from build123d import *

# Parameters (mm, degrees)
EXTRUDE_1_DEPTH     = 2
SKETCH_2_R          = 2
EXTRUDE_2_DEPTH     = 7
CUT_EXTRUDE_2_DEPTH = 10


with BuildPart() as part:
    # 草图1 → 凸台-拉伸1 (new body)
    with BuildSketch(Plane(origin=(0, 0, 0), x_dir=(1, 0, 0), z_dir=(0, 1, 0))):
        with BuildLine():
            Line((-65, 5), (15, 5))
            ThreePointArc((15, 5), (20, 0), (15, -5))
            Line((15, -5), (-65, -5))
            ThreePointArc((-65, -5), (-70, 0), (-65, 5))
        make_face()
    extrude(amount=EXTRUDE_1_DEPTH)

    # 草图2 → 凸台-拉伸2 (add)
    with BuildSketch(Plane(origin=(0, 2, 0), x_dir=(1, 0, 0), z_dir=(0, 1, 0))):
        with Locations((15, 0)):
            Circle(SKETCH_2_R)
        with BuildLine():
            ThreePointArc((-63, 0), (-63.585786438, 1.414213562), (-65, 2))
            Line((-65, 2), (-65, -2))
            ThreePointArc((-65, -2), (-63.585786438, -1.414213562), (-63, 0))
        make_face()
        with BuildLine():
            Line((-65, -2), (-65, 2))
            ThreePointArc((-65, 2), (-67, 0), (-65, -2))
        make_face()
    extrude(amount=EXTRUDE_2_DEPTH)

    # 草图4 → 切除-拉伸2 (cut)
    with BuildSketch(Plane.XZ):
        with BuildLine():
            ThreePointArc((-23.015444247, 0.248069469), (-25.248069469, 1.984555753), (-26.984555753, -0.248069469))
            Line((-26.984555753, -0.248069469), (-23.015444247, 0.248069469))
        make_face()
        with BuildLine():
            Line((-23.015444247, 0.248069469), (-26.984555753, -0.248069469))
            ThreePointArc((-26.984555753, -0.248069469), (-24.875725117, -1.996135204), (-23, 0))
            ThreePointArc((-23, 0), (-23.003864796, 0.124274883), (-23.015444247, 0.248069469))
        make_face()
    extrude(amount=-CUT_EXTRUDE_2_DEPTH, mode=Mode.SUBTRACT)


solid = part.part
Build history of the part. All positions in model axes, mm. Coordinates: 2 decimals unless noted, no trailing zeros. Write each loop counter-clockwise with the first axis right and the second up, starting at its lowest first coordinate (ties: lowest second). Pieces come first, ordered by that corner, then holes.
(1) Pin check, flat tips, straight feed: pin 1 Ø2 at (x, y) = (-54.5, 3.5) entering from -Z; pin 2 Ø3 at (x, z) = (-30.5, 2.5) entering from +Y. Stop position of each tip, or through.
(2) Cut at B-B on y = 3.25. List the corners of the cut face in (x, z), and give its area (3 significant figures).
(3) Cut at A-A on x = -25. List the corners of the cut face in (y, z).
(4) Cut at C-C on x = -54. List the corners of the cut face in (y, z), and give its area (3 significant figures).
(5) Mould opens along X. For faces 1 (the flat face through (-65, 9, 0)), 2 (the cylindrical face through (20, 1, 0)), 3 (the cylindrical face through (13.4, 5.5, 1.2)) say: pulls with the +X half, pulls with the -X half, needs draft (parallel to the pull), parting line crosses it, or undercut.
(6) Cut at D-D on z = 4.25. List the corners of the cut face in (x, y), and give its area (3 significant figures).
(7) Drill centre lines: line 1 (Y direction, x = -29, z = -1.25); line 2 (X direction, y = 3, z = -1.75); line 3 (Z direction, x = 13.5, y = 2.5). Where is each one in solid material? Low to high.
Working result:
1. pin 1: passes through
1. pin 2: stops at y = 2
2. outline: circle Ø4 at (-65, 0); circle Ø4 at (15, 0)
2. area: 25.1 mm2
3. outline: (0, -5) - (2, -5) - (2, -2) - (0, -2) - close; (0, 2) - (2, 2) - (2, 5) - (0, 5) - close
4. outline: (0, -5) - (2, -5) - (2, 5) - (0, 5) - close
4. area: 20.0 mm2
5. face 1: needs draft
5. face 2: pulls with the +X half
5. face 3: undercut
6. outline: (-67.63, 0) - (17.63, 0) - (17.63, 2) - (-67.63, 2) - close
6. area: 171 mm2
7. line 1: y = 0 to 2
7. line 2: x = -65.97 to -64.03, 14.03 to 15.97
7. line 3: z = -1.32 to 1.32
